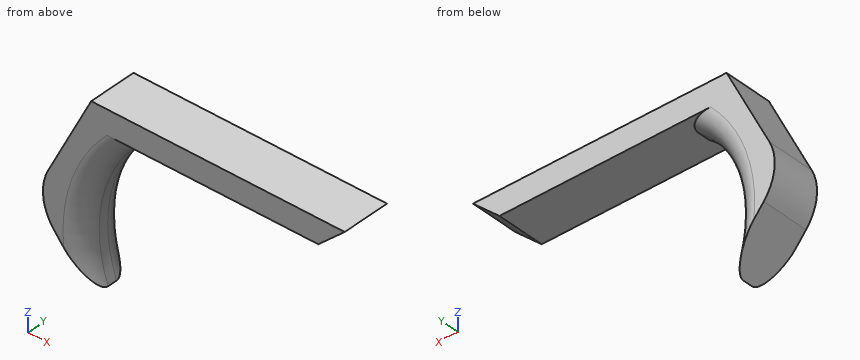
```python
from build123d import *

# Parameters (mm, degrees)
F1_DEPTH = 12.7
F2_R     = 5.08


with BuildPart() as f1:
    # F0 (on Front) → F1 (new body)
    with BuildSketch(Plane.XZ):
        with BuildLine():
            Line((66.802, 0), (0, 0))
            Line((0, 0), (-11.343573, -22.384649))
            ThreePointArc((-11.343573, -22.384649), (-12.637739, -29.525329), (-9.810389, -36.20891))
            Line((-9.810389, -36.20891), (0, -48.09675))
            ThreePointArc((0, -48.09675), (-0.98103, -25.294337), (11.747858, -6.35))
            Line((11.747858, -6.35), (59.844611, -6.35))
            Line((59.844611, -6.35), (66.802, 0))
        make_face()
    extrude(amount=F1_DEPTH)

    # F2
    f2_edges = [f1.edges().sort_by_distance(p)[0] for p in [
        (-0.98103, -12.7, -25.294337),
        (-0.98103, 0, -25.294337),
    ]]
    fillet(f2_edges, radius=F2_R)


solid = f1.part
```
Design review of the part built by this model. Coordinates are the model's own, in mm. Round coordinates to 2 decimals unless told otherwise and drop trailing zeros. Write each loop counter-clockwise with the first axis right and the second up, starting at its lowest first coordinate (ties: lowest second). Pieces come first, ordered by that corner, then holes.
Item 1: We need section C-C on y = -1.25. Write out the cut boundary in (x, z).
Item 2: We need section B-B on x = 56. Write out the cut boundary in (y, z), and give its area (3 significant figures).
Item 3: For probe 1 along Z at (x, y) = (50.5, -7.25); probe 2 along X at (y, z) = (-2.25, -45.5); probe 3 along X at (y, z) = (-9, -29), list the stretches that pass through material, from the lowest coordinate up.
Item 4: We need section A-A on y = -6.75. Write out the cut boundary in (x, z), and give its area (3 significant figures).
Item 5: Clearance check with flat-ended pins moving along their axes: pin 1 Ø3 at (y, z) = (-5, -14) entering from -X; pin 2 Ø5 at (y, z) = (-2.5, -34.5) entering from +X; pin 3 Ø2 at (y, z) = (-10, -36) entering from +X; pin 4 Ø4 at (x, y) = (39.5, -4.5) entering from +Z. State where each tip first meets the part, or that it passes through.
Returned:
1. outline: (-11.34, -22.38) arc R12.7 ccw to (-9.81, -36.21) - (-2.94, -44.54) arc R38.32 cw to (9.01, -6.35) - (59.84, -6.35) - (66.8, 0) - (0, 0) - close
2. outline: (-12.7, -6.35) - (0, -6.35) - (0, 0) - (-12.7, 0) - close
2. area: 80.6 mm2
3. probe 1: z = -6.35 to 0
3. probe 2: x = -2.14 to -1.77
3. probe 3: x = -12.68 to -2.01
4. outline: (-11.34, -22.38) arc R12.7 ccw to (-9.81, -36.21) - (0, -48.1) arc R36.57 cw to (11.75, -6.35) - (59.84, -6.35) - (66.8, 0) - (0, 0) - close
4. area: 788 mm2
5. pin 1: stops at x = -7.85
5. pin 2: stops at x = -2.31
5. pin 3: stops at x = -2.53
5. pin 4: stops at z = 0
